Source: CAD feature listing. Evaluate the final solid. Frame: model axes, mm. A direction names the side the tool comes from. Round coordinates to 2 decimals unless told otherwise and drop trailing zeros. Loops run counter-clockwise (first coordinate to the right, second up) from the corner with the lowest first, then second, coordinate; pieces in that order, holes last. Notation, with made-up numbers: (84.25, 54) -> (97.25, 54) arc R11 cw to (97.25, 68) -> close; hole circle Ø3 at (14, -35). An arc over 180 degrees is marked (long way). Write item = value, one per line.
from build123d import *

# Parameters (mm, degrees)
BOSS_EXTRUDE1_DEPTH = 38
FILLET2_R           = 7


with BuildPart() as part:
    # Sketch1 → Boss-Extrude1 (new body)
    with BuildSketch(Plane(origin=(0, 0, 0), x_dir=(1, 0, 0), z_dir=(0, 1, 0))):
        Polygon((0, 0), (0, 46), (6, 46), (6, 4), (34.5, 4), (34.5, 0), align=None)
    extrude(amount=BOSS_EXTRUDE1_DEPTH)

    # Fillet2
    fillet2_edges = [part.edges().sort_by_distance(p)[0] for p in [
        (6, 19, -4),
        (3, 38, -46),
        (3, 0, -46),
        (34.5, 0, -2),
        (34.5, 38, -2),
    ]]
    fillet(fillet2_edges, radius=FILLET2_R)


solid = part.part
1. Section query C-C (z = -16.5). Return the cut outline in (x, y).
Evaluation:
outline = (0, 0) -> (6, 0) -> (6, 38) -> (0, 38) -> close
2. Section query B-B (x = 20.5). Return the cut outline in (y, z), then the cut area to 3 significant figures.
Evaluation:
outline = (0, -4) -> (38, -4) -> (38, 0) -> (0, 0) -> close
area = 152 mm²
3. Set-up query: faces 1 (the face through (6, 19, -29)), 2 (the face through (34.5, 19, -2)). Return all of +Z, -Z, +X, -X, +Y, -Y with unobstructed straight access to the full face (end or side cutting, diameter ignored); none if empty.
Evaluation:
face_1 = -Z, +X, +Y, -Y
face_2 = +Z, -Z, +X, +Y, -Y
4. Contact query for flat-ended pins moving along their axis: pin 1 Ø8 at (x, y) = (30.5, 26.5) entering from -Z; pin 2 Ø4 at (y, z) = (11, -31) entering from +X. Output: stop coordinate, or through.
Evaluation:
pin_1 = -4
pin_2 = 6
5. Section query D-D (y = 35.5). Return the cut outline in (x, z), then the cut area to 3 significant figures.
Evaluation:
outline = (0, -44.36) -> (6, -44.36) -> (6, -11) arc R7 cw to (13, -4) -> (32.86, -4) -> (32.86, 0) -> (0, 0) -> close
area = 384 mm²
6. Line query: probe 1 along Z at (x, y) = (30, 11); probe 2 along X at (y, z) = (9, -13); probe 3 along X at (y, z) = (20, -9.5). Output: solid intervals per line, ascending. Write a range as from..to.
Evaluation:
probe_1 = -4..0
probe_2 = 0..6
probe_3 = 0..6.16
7. Section query A-A (y = 27). Return the cut outline in (x, z), then the cut area to 3 significant figures.
Evaluation:
outline = (0, -46) -> (6, -46) -> (6, -11) arc R7 cw to (13, -4) -> (34.5, -4) -> (34.5, 0) -> (0, 0) -> close
area = 401 mm²
